from build123d import *

# Parameters (mm, degrees)
F1_DEPTH  = 1.5
F3_DEPTH  = 63
F6_DEPTH  = 68
F8_W      = 5.6641247272
F8_H      = 11.9948398471
F9_DEPTH  = 0.5
F10_W     = 1.7004162073
F10_H     = 6.2374770641
F11_DEPTH = 2
F13_DEPTH = 3


with BuildPart() as f1:
    # F0 (on Front) → F1 (new body, symmetric)
    with BuildSketch(Plane.XZ):
        with BuildLine():
            Line((53, -51.5), (58, -51.5))
            ThreePointArc((58, -51.5), (61.5355339059, -50.0355339059), (63, -46.5))
            Line((63, -46.5), (63, 46.5))
            ThreePointArc((63, 46.5), (61.5355339059, 50.0355339059), (58, 51.5))
            Line((58, 51.5), (-58, 51.5))
            ThreePointArc((-58, 51.5), (-61.5355339059, 50.0355339059), (-63, 46.5))
            Line((-63, 46.5), (-63, -46.5))
            ThreePointArc((-63, -46.5), (-61.5355339059, -50.0355339059), (-58, -51.5))
            Line((-58, -51.5), (-53, -51.5))
            ThreePointArc((-53, -51.5), (-49.4644660941, -50.0355339059), (-48, -46.5))
            Line((-48, -46.5), (-48, -13.5))
            ThreePointArc((-48, -13.5), (-39.2132034356, 7.7132034356), (-18, 16.5))
            Line((-18, 16.5), (18, 16.5))
            ThreePointArc((18, 16.5), (39.2132034356, 7.7132034356), (48, -13.5))
            Line((48, -13.5), (48, -46.5))
            ThreePointArc((48, -46.5), (49.4644660941, -50.0355339059), (53, -51.5))
        make_face()
    extrude(amount=F1_DEPTH, both=True)

    # F2 (on Right) → F3 (join, symmetric)
    with BuildSketch(Plane.YZ):
        with BuildLine():
            Line((0, 21.5), (0, 51.5))
            Line((0, 51.5), (-15, 51.5))
            ThreePointArc((-15, 51.5), (-25.6066017178, 47.1066017178), (-30, 36.5))
            ThreePointArc((-30, 36.5), (-25.6066017178, 25.8933982822), (-15, 21.5))
            Line((-15, 21.5), (0, 21.5))
        make_face()
    extrude(amount=F3_DEPTH, both=True)

    # F5 (on face) → F6 (join)
    with BuildSketch(Plane(origin=(0, 0, 21.5), x_dir=(1, 0, 0), z_dir=(0, 0, -1))):
        Polygon((-48, 15), (-63, 15), (-63, 1.5), (-59, 1.5), (-59, 12.5), (-48, 12.5), align=None)
    extrude(amount=F6_DEPTH)

    # F7: F1 across plane


with BuildPart() as f1_1:
    add(f1.part)
    add(f1.part.mirror(Plane.YZ))

    # F8 (on face) → F9 (join)
    with BuildSketch(Plane.XZ.offset(1.5)):
        with Locations((-56.1679376364, 15.5025800765)):
            Rectangle(F8_W, F8_H)
    extrude(amount=F9_DEPTH)

    # F10 (on face) → F11 (join)
    with BuildSketch(Plane.XZ.offset(2)):
        with Locations((-56.6318407655, 17.4285247922)):
            Rectangle(F10_W, F10_H)
    extrude(amount=F11_DEPTH)

    # F12 (on face) → F13 (cut)
    with BuildSketch(Plane.YZ.offset(-55.7816326618)):
        Polygon((-2, 14.3097862601), (-4, 20.5472633243), (-4, 14.3097862601), align=None)
    extrude(amount=-F13_DEPTH, mode=Mode.SUBTRACT)


solid = f1_1.part
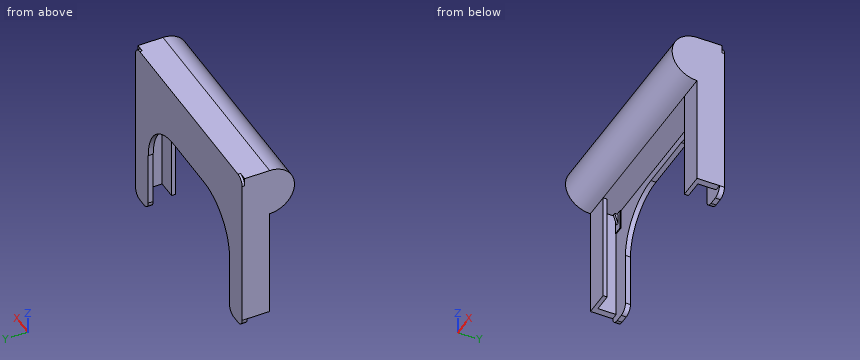
The listing builds one solid part. Answer for the finished solid, in the listing's coordinates (mm). Round coordinates to 2 decimals unless told otherwise and drop trailing zeros. Write each loop counter-clockwise with the first axis right and the second up, starting at its lowest first coordinate (ties: lowest second). Pieces come first, ordered by that corner, then holes. Notation, with made-up numbers: M 78,-33.75 L 85,-33.75 A30 ccw 85,5.25 Z; hole C 87.5,45 d4. An arc over 180 degrees is marked long. Write each question's results on one line, items separated by ' | '. Start each with the question number.
Item 1: Find section D-D on z = 24.5. Write down the section's boundary in (x, y).
Item 2: Straight lines are drawn through the part: probe 1 along X at (y, z) = (-13.5, -9); probe 2 along X at (y, z) = (-7.5, -19.5); probe 3 along Z at (x, y) = (39, -7). For each, find the intervals that lie inside material, in ascending order.
Item 3: Given pin 1 Ø1.7 at (x, z) = (-56, 16) entering from -Y; pin 2 Ø2 at (x, y) = (44.5, -20.5) entering from -Z; pin 3 Ø2.5 at (x, y) = (3, -0.5) entering from -Z, each flat-ended and moving along its own axis, determine where each tip first touches the part or whether it passes through.
Item 4: Find section A-A on z = -44.5. Write down the section's boundary in (x, y), and give its area (3 significant figures).
Item 5: Find section C-C on y = -27. Write down the section's boundary in (x, z).
Item 6: Find section B-B on x = 10.5. Write down the section's boundary in (y, z), and give its area (3 significant figures).
Answer block:
1) outline: M -63,-24 L 63,-24 L 63,1.5 L -63,1.5 Z
2) probe 1: x = -63 to -48, 48 to 63 | probe 2: x = -63 to -59, 59 to 63 | probe 3: z = 21.5 to 51.5
3) pin 1: stops at y = -15 | pin 2: stops at z = 22.19 | pin 3: stops at z = 16.5
4) outline: M -63,-15 L -48,-15 L -48,-12.5 L -59,-12.5 L -59,-1.5 L -48,-1.5 L -48,1.5 L -63,1.5 Z; M 48,-15 L 63,-15 L 63,1.5 L 48,1.5 L 48,-1.5 L 59,-1.5 L 59,-12.5 L 48,-12.5 Z | area: 253 mm²
5) outline: M -63,27.5 L 63,27.5 L 63,45.5 L -63,45.5 Z
6) outline: M -15,21.5 L -1.5,21.5 L -1.5,16.5 L 1.5,16.5 L 1.5,51.5 L -15,51.5 A15 ccw Z | area: 863 mm²
